The model under review builds one solid part; all positions refer to its coordinate system, in mm. A direction names the side the tool comes from. Coordinates: 2 decimals unless noted, no trailing zeros. Order: outer loops, then holes, each group sorted by start corner. A loop starts at its lowest first (then second) coordinate and runs counter-clockwise, first axis right, second up. Notation, with made-up numbers: (71, 22) - (107, 22) arc R22 cw to (107, 48) - close; hole circle Ø9 at (16.5, 6). An arc over 180 degrees is marked (long way). Answer in a Markdown table with one row per item.
```python
from build123d import *

# Parameters (mm, degrees)
ESBO_O1_W                = 92
ESBO_O1_H                = 26
RESSALTO_EXTRUS_O1_DEPTH = 26.2
ESBO_O2_W                = 16.5
ESBO_O2_H                = 10
CORTE_EXTRUS_O1_DEPTH    = 27
ESBO_O3_R                = 2.5
CORTE_EXTRUS_O2_DEPTH    = 27.2
ESBO_O4_R                = 2.85
RESSALTO_EXTRUS_O2_DEPTH = 17.5


with BuildPart() as part:
    # Esboço1 → Ressalto-extrusão1 (new body)
    with BuildSketch(Plane.XY):
        Rectangle(ESBO_O1_W, ESBO_O1_H)
    extrude(amount=RESSALTO_EXTRUS_O1_DEPTH)

    # Esboço2 → Corte-extrusão1 (cut, through all)
    with BuildSketch(Plane.XZ.offset(13)):
        with Locations((-32.75, 21.2)):
            Rectangle(ESBO_O2_W, ESBO_O2_H)
        with Locations((0, 21.2)):
            Rectangle(ESBO_O2_W, ESBO_O2_H)
        with Locations((32.75, 21.2)):
            Rectangle(ESBO_O2_W, ESBO_O2_H)
    extrude(amount=-CORTE_EXTRUS_O1_DEPTH, mode=Mode.SUBTRACT)

    # Esboço3 → Corte-extrusão2 (cut, through all)
    with BuildSketch(Plane(origin=(0, 0, 0), x_dir=(-1, 0, 0), z_dir=(0, 0, -1))):
        with Locations((-15.9, 4)):
            Circle(ESBO_O3_R)
        with Locations((15.9, 4)):
            Circle(ESBO_O3_R)
    extrude(amount=-CORTE_EXTRUS_O2_DEPTH, mode=Mode.SUBTRACT)

    # Esboço4 → Ressalto-extrusão2 (add)
    with BuildSketch(Plane.XY.offset(16.2)):
        with Locations((0, -5.85)):
            Circle(ESBO_O4_R)
        with Locations((32.75, -5.85)):
            Circle(ESBO_O4_R)
        with Locations((-32.75, -5.85)):
            Circle(ESBO_O4_R)
    extrude(amount=RESSALTO_EXTRUS_O2_DEPTH)


solid = part.part
```
Item 1: We need section D-D, the plane x = 32.75. Write out the cut boundary in (y, z).
Check values:
| item | result |
|---|---|
| outline | (-13, 0) - (13, 0) - (13, 16.2) - (-3, 16.2) - (-3, 33.7) - (-8.7, 33.7) - (-8.7, 16.2) - (-13, 16.2) - close |
Item 2: Mouldability with a two-part tool opening along X and no side actions: class faces 1 (the face through (46, 0, 13)), 2 (the face through (-1, 13, 10)), 3 (the face through (-46, 0, 13)), 4 (the face through (41, 0, 21)) as +X half, -X half, draft (parallel to the pull), parting line (faces both ways), or undercut.
Check values:
| item | result |
|---|---|
| face 1 | +X half |
| face 2 | draft |
| face 3 | -X half |
| face 4 | undercut |
Item 3: We need section B-B, the plane y = 4. Write out the cut boundary in (x, z).
Check values:
| item | result |
|---|---|
| outline | (-46, 0) - (-18.4, 0) - (-18.4, 26.2) - (-24.5, 26.2) - (-24.5, 16.2) - (-41, 16.2) - (-41, 26.2) - (-46, 26.2) - close; (-13.4, 0) - (13.4, 0) - (13.4, 26.2) - (8.25, 26.2) - (8.25, 16.2) - (-8.25, 16.2) - (-8.25, 26.2) - (-13.4, 26.2) - close; (18.4, 0) - (46, 0) - (46, 26.2) - (41, 26.2) - (41, 16.2) - (24.5, 16.2) - (24.5, 26.2) - (18.4, 26.2) - close |
Item 4: Clearance check with flat-ended pins moving along their axes: pin 1 Ø3 at (x, y) = (17, -7) entering from -Z; pin 2 Ø2 at (x, y) = (-7, 1.5) entering from +Z; pin 3 Ø5 at (x, y) = (-17.5, 6) entering from +Z. State where each tip first meets the part, or that it passes through.
Check values:
| item | result |
|---|---|
| pin 1 | z = 0 |
| pin 2 | z = 16.2 |
| pin 3 | z = 26.2 |
Item 5: Tool access review of faces 5 (the face through (16, 0, 26.2)), 6 (the face through (-30.1, -6.9, 24.8)), 7 (the face through (16.23, 6.48, 12.92)): name each direction out of +Z, -Z, +X, -X, +Y, -Y from which nothing blocks a thin tool from reaching the whole face with its end or side.
Check values:
| item | result |
|---|---|
| face 5 | +Z, +Y, -Y |
| face 6 | +Z |
| face 7 | +Z, -Z |
Item 6: We need section A-A, the plane x = -15.9. Write out the cut boundary in (y, z), then the cut area to 3 significant figures.
Check values:
| item | result |
|---|---|
| outline | (-13, 0) - (1.5, 0) - (1.5, 26.2) - (-13, 26.2) - close; (6.5, 0) - (13, 0) - (13, 26.2) - (6.5, 26.2) - close |
| area | 550 mm^2 |
Item 7: To check wall thickness, follow line 1 (X direction, y = 4.25, z = 12.5); line 2 (Y direction, x = -15.9, z = 19.5); line 3 (X direction, y = 4.5, z = 23). State the ranges of each line that lie inside material, in increasing order. Write a range as from..to.
Check values:
| item | result |
|---|---|
| line 1 | -46..-18.39, -13.41..13.41, 18.39..46 |
| line 2 | -13..1.5, 6.5..13 |
| line 3 | -46..-41, -24.5..-18.35, -13.45..-8.25, 8.25..13.45, 18.35..24.5, 41..46 |
Item 8: We need section C-C, the plane y = -11. Write out the cut boundary in (x, z), then the cut area to 3 significant figures.
Check values:
| item | result |
|---|---|
| outline | (-46, 0) - (46, 0) - (46, 26.2) - (41, 26.2) - (41, 16.2) - (24.5, 16.2) - (24.5, 26.2) - (8.25, 26.2) - (8.25, 16.2) - (-8.25, 16.2) - (-8.25, 26.2) - (-24.5, 26.2) - (-24.5, 16.2) - (-41, 16.2) - (-41, 26.2) - (-46, 26.2) - close |
| area | 1,920 mm^2 |
